Here's the drawing with two shaded views (mm, measured from the low corner). I have some questions. Round coordinates to 2 decimals unless told otherwise and drop trailing zeros. Order: outer loops, then holes, each group sorted by start corner. A loop starts at its lowest first (then second) coordinate and runs counter-clockwise, first axis right, second up. Notation, with made-up numbers: (85, -38) - (130, -38) arc R33 cw to (130, -6) - close; hole circle Ø10 at (40.5, -36). An arc over 180 degrees is marked (long way). One line per item, written item: value.
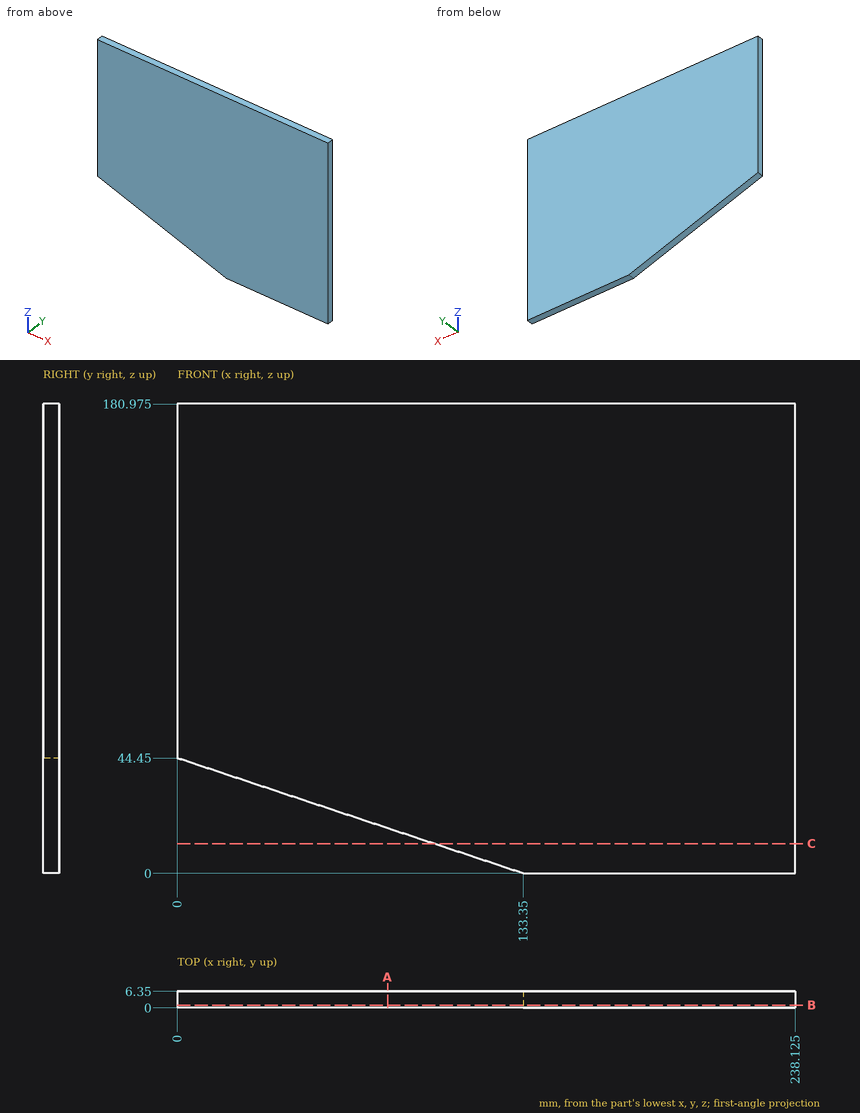
Q1. If we section it at B-B, the plane y = 1: Please give me the cut outline in (x, z) (3 decimals), then the cut area to 3 significant figures.
Results list:
outline: (0, 44.45) - (133.35, 0) - (238.125, 0) - (238.125, 180.975) - (0, 180.975) - close
area: 40,100 mm²
Q2. If we section it at A-A, the plane x = 81: Please give me the cut outline in (y, z) (3 decimals).
Results list:
outline: (0, 17.45) - (6.35, 17.45) - (6.35, 180.975) - (0, 180.975) - close
Q3. If I drill on line 1 along Z through (x, y) = (14.5, 5.25) (3 decimals); line 2 along Z through (x, y) = (108, 5) (3 decimals), over which ranges is the centre line in solid material (lowest first)?
Results list:
line 1: 39.617 to 180.975
line 2: 8.45 to 180.975
Q4. If we section it at C-C, the plane z = 11.5: Please give me the cut outline in (x, y) (3 decimals), then the cut area to 3 significant figures.
Results list:
outline: (98.85, 0) - (238.125, 0) - (238.125, 6.35) - (98.85, 6.35) - close
area: 884 mm²
